The figure shows three views and two pictorial views of one solid part (mm, origin at its lowest corner). Answer the questions. A direction names the side the tool comes from. Coordinates: 2 decimals unless noted, no trailing zeros. Write each loop counter-clockwise with the first axis right and the second up, starting at its lowest first coordinate (ties: lowest second). Pieces come first, ordered by that corner, then holes.
Item 1: Each of these flat-tipped pins is pushed along its axis until it touches: P1, Ø1.6, axis at y = 15.5, z = 6.5, coming from the +X side; P2, Ø3, axis at x = 4, z = 11, coming from the +Y side; P3, Ø6, axis at x = 7.5, y = 5, coming from the -Z side; P4, Ø0.6, axis at x = 8, y = 15.5, coming from the +Z side. Where does it stop, or does it pass through?
Item 2: Section B-B (z = 14.5) is taken. Give the vertices of the cut face in (x, y), then the cut area to 3 significant figures.
Item 3: Straight lines are drawn through the part: probe 1 along Z at (x, y) = (4, 2.5); probe 2 along Z at (x, y) = (6.75, 15); probe 3 along X at (y, z) = (6.75, 2.25). For each, find the intervals that lie inside material, in ascending order.
Item 4: Determine the mould class of the marked faces 1, 2 and 3 for opening direction X: released by +X, released by -X, zero draft, split by the parting line, or undercut.
Item 5: Section A-A (x = 10) is taken. Give the vertices of the cut face in (y, z).
Item 6: A tool of negligible diameter and unlimited length cuts with its end or side. For the marked faces 4 and 5, from which of +Z, -Z, +X, -X, +Y, -Y can it reach the whole face along a straight path? Write none if from no direction.
Item 7: Section C-C (y = 5.25) is taken. Give the vertices of the cut face in (x, z), then the cut area to 3 significant figures.
Item 8: Section D-D (x = 1) is taken. Give the vertices of the cut face in (y, z), then the cut area to 3 significant figures.
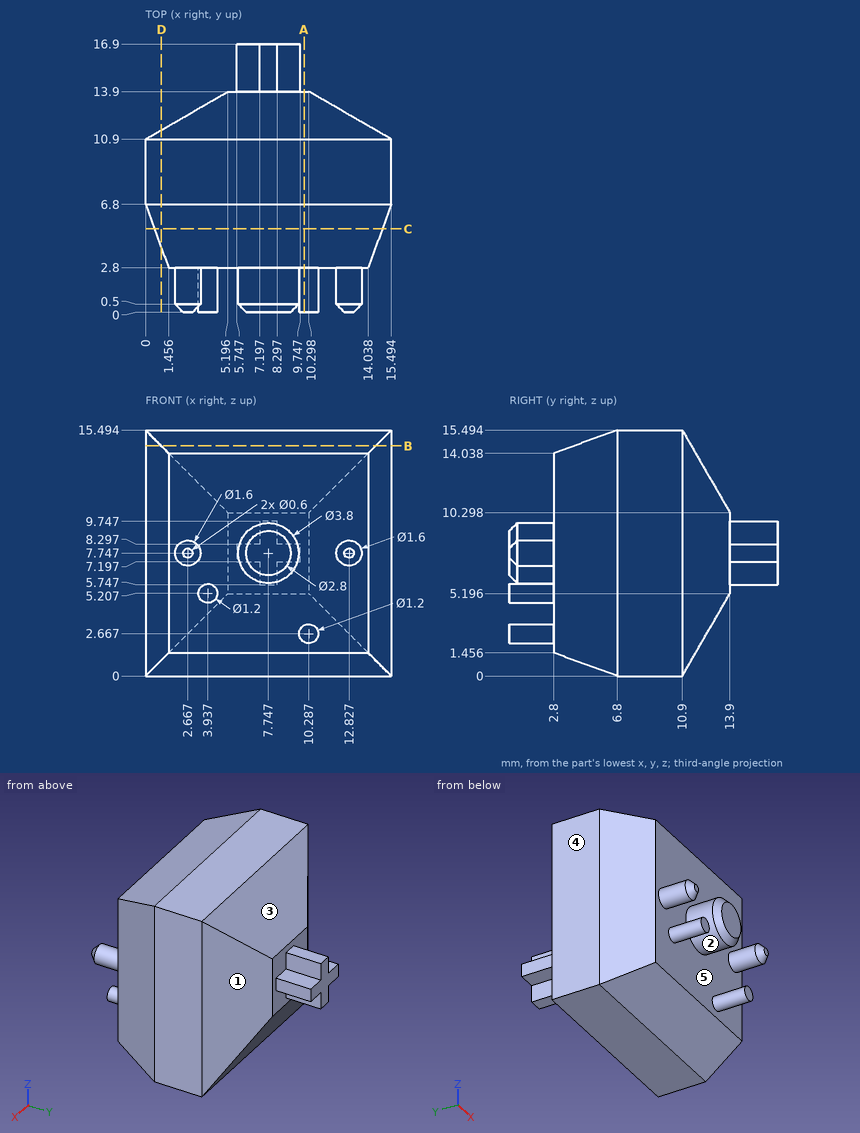
Established:
1. P1: stops at x = 9.75
1. P2: stops at y = 13.9
1. P3: stops at z = 0
1. P4: stops at z = 9.75
2. outline: (0, 6.8) - (0.99, 4.07) - (14.5, 4.07) - (15.49, 6.8) - (15.49, 10.9) - (14.5, 11.47) - (0.99, 11.47) - (0, 10.9) - close
2. area: 111 mm2
3. probe 1: z = 4.61 to 5.8
3. probe 2: z = 7.2 to 8.3
3. probe 3: x = 0.02 to 15.48
4. face 1: released by +X
4. face 2: undercut
4. face 3: zero draft
5. outline: (0, 2.14) - (2.8, 2.14) - (2.8, 1.46) - (6.8, 0) - (10.9, 0) - (13.9, 5.2) - (13.9, 10.3) - (10.9, 15.49) - (6.8, 15.49) - (2.8, 14.04) - (2.8, 3.19) - (0, 3.19) - close
6. face 4: +Z, -Z, -X, +Y, -Y
6. face 5: -Y
7. outline: (0.56, 0.56) - (14.93, 0.56) - (14.93, 14.93) - (0.56, 14.93) - close
7. area: 206 mm2
8. outline: (4.05, 1) - (6.8, 0) - (10.9, 0) - (11.48, 1) - (11.48, 14.49) - (10.9, 15.49) - (6.8, 15.49) - (4.05, 14.49) - close
8. area: 112 mm2
